Can you work these out from the model? Positions are in its coordinate system, mm. A direction names the side the tool comes from. Coordinates: 2 decimals unless noted, no trailing zeros. Loops run counter-clockwise (first coordinate to the right, second up) from the corner with the lowest first, then second, coordinate; pieces in that order, holes last.
```python
from build123d import *

# Parameters (mm, degrees)
SKETCH1_R           = 1.5
SKETCH1_R_2         = 18
BOSS_EXTRUDE1_DEPTH = 2
SKETCH1_3_R         = 31
SKETCH1_3_R_2       = 25
BOSS_EXTRUDE2_DEPTH = 1


with BuildPart() as part:
    # Sketch1 → Boss-Extrude1 (new body)
    with BuildSketch(Plane(origin=(0, 0, 0), x_dir=(1, 0, 0), z_dir=(0, 1, 0))):
        with BuildLine():
            ThreePointArc((33.442622951, 6.131147541), (24.04163056, 24.04163056), (6.131147541, 33.442622951))
            ThreePointArc((6.131147541, 33.442622951), (4.602624673, 34.335520561), (4, 36))
            ThreePointArc((4, 36), (0, 40), (-4, 36))
            ThreePointArc((-4, 36), (-4.602624673, 34.335520561), (-6.131147541, 33.442622951))
            ThreePointArc((-6.131147541, 33.442622951), (-24.04163056, 24.04163056), (-33.442622951, 6.131147541))
            ThreePointArc((-33.442622951, 6.131147541), (-34.335520561, 4.602624673), (-36, 4))
            ThreePointArc((-36, 4), (-40, 0), (-36, -4))
            ThreePointArc((-36, -4), (-34.335520561, -4.602624673), (-33.442622951, -6.131147541))
            ThreePointArc((-33.442622951, -6.131147541), (-24.04163056, -24.04163056), (-6.131147541, -33.442622951))
            ThreePointArc((-6.131147541, -33.442622951), (-4.602624673, -34.335520561), (-4, -36))
            ThreePointArc((-4, -36), (0, -40), (4, -36))
            ThreePointArc((4, -36), (4.602624673, -34.335520561), (6.131147541, -33.442622951))
            ThreePointArc((6.131147541, -33.442622951), (24.04163056, -24.04163056), (33.442622951, -6.131147541))
            ThreePointArc((33.442622951, -6.131147541), (34.335520561, -4.602624673), (36, -4))
            ThreePointArc((36, -4), (40, 0), (36, 4))
            ThreePointArc((36, 4), (34.335520561, 4.602624673), (33.442622951, 6.131147541))
        make_face()
        with Locations((36, 0)):
            Circle(SKETCH1_R, mode=Mode.SUBTRACT)
        with Locations((0, -36)):
            Circle(SKETCH1_R, mode=Mode.SUBTRACT)
        with Locations((0, 36)):
            Circle(SKETCH1_R, mode=Mode.SUBTRACT)
        with Locations((-36, 0)):
            Circle(SKETCH1_R, mode=Mode.SUBTRACT)
        Circle(SKETCH1_R_2, mode=Mode.SUBTRACT)
    extrude(amount=BOSS_EXTRUDE1_DEPTH)

    # Sketch1<3> → Boss-Extrude2 (add)
    with BuildSketch(Plane(origin=(0, 0, 0), x_dir=(1, 0, 0), z_dir=(0, 1, 0))):
        Circle(SKETCH1_3_R)
        Circle(SKETCH1_3_R_2, mode=Mode.SUBTRACT)
    extrude(amount=-BOSS_EXTRUDE2_DEPTH)


solid = part.part
```
(1) I want a section at D-D on z = -12. Write out the boundary of the cut face in (x, y).
Check values:
outline: (-31.81, 0) - (-28.58, 0) - (-28.58, -1) - (-21.93, -1) - (-21.93, 0) - (-13.42, 0) - (-13.42, 2) - (-31.81, 2) - close; (13.42, 0) - (21.93, 0) - (21.93, -1) - (28.58, -1) - (28.58, 0) - (31.81, 0) - (31.81, 2) - (13.42, 2) - close
(2) I'm going to push flat-ended pins straight in: pin 1 (1.5 mm diameter, centred on x = 17.5, y = 1.5, fed in from -Z); pin 2 (5 mm diameter, centred on x = 0, z = 36, fed in from -Y). Where does each tip first touch, or does it pass through?
Check values:
pin 1: stops at z = -29.59
pin 2: stops at y = 0
(3) I want a section at B-B on z = 0. Write out the boundary of the cut face in (x, y), then the cut area to 3 significant figures.
Check values:
outline: (-40, 0) - (-37.5, 0) - (-37.5, 2) - (-40, 2) - close; (-34.5, 0) - (-31, 0) - (-31, -1) - (-25, -1) - (-25, 0) - (-18, 0) - (-18, 2) - (-34.5, 2) - close; (18, 0) - (25, 0) - (25, -1) - (31, -1) - (31, 0) - (34.5, 0) - (34.5, 2) - (18, 2) - close; (37.5, 0) - (40, 0) - (40, 2) - (37.5, 2) - close
area: 88.0 mm2
(4) If I drill on probe 1 along Z at (x, y) = (0, 1.45); probe 2 along Z at (x, y) = (36, 0.65), over which ranges is the centre line in solid material (lowest first)?
Check values:
probe 1: z = -40 to -37.5, -34.5 to -18, 18 to 34.5, 37.5 to 40
probe 2: z = -4 to -1.5, 1.5 to 4
(5) I want a section at A-A on x = 0. Write out the boundary of the cut face in (y, z).
Check values:
outline: (-1, -31) - (0, -31) - (0, -34.5) - (2, -34.5) - (2, -18) - (0, -18) - (0, -25) - (-1, -25) - close; (-1, 25) - (0, 25) - (0, 18) - (2, 18) - (2, 34.5) - (0, 34.5) - (0, 31) - (-1, 31) - close; (0, -40) - (2, -40) - (2, -37.5) - (0, -37.5) - close; (0, 37.5) - (2, 37.5) - (2, 40) - (0, 40) - close
(6) I want a section at C-C on y = 1.1. Write out the boundary of the cut face in (x, z), then the cut area to 3 significant figures.
Check values:
outline: (-36, -4) arc R2.6 cw to (-33.44, -6.13) arc R34 ccw to (-6.13, -33.44) arc R2.6 cw to (-4, -36) arc R4 ccw to (4, -36) arc R2.6 cw to (6.13, -33.44) arc R34 ccw to (33.44, -6.13) arc R2.6 cw to (36, -4) arc R4 ccw to (36, 4) arc R2.6 cw to (33.44, 6.13) arc R34 ccw to (6.13, 33.44) arc R2.6 cw to (4, 36) arc R4 ccw to (-4, 36) arc R2.6 cw to (-6.13, 33.44) arc R34 ccw to (-33.44, 6.13) arc R2.6 cw to (-36, 4) arc R4 ccw to start; hole circle Ø3 at (-36, 0); hole circle Ø36 at (0, 0); hole circle Ø3 at (0, -36); hole circle Ø3 at (0, 36); hole circle Ø3 at (36, 0)
area: 2,760 mm2
(7) Which directions (+Z, -Z, +X, -X, +Y, -Y) give clear straight access to the entire face, cutting with the end or side of a thin tool? Please do faces 1 (the flat face through (11, 0, 16)), 2 (the flat face through (-0.6, 2, -18.3)).
Check values:
face 1: -Y
face 2: +Z, -Z, +X, -X, +Y
(8) If we mould it in two halves opening along X, with no side actions, what happens to faces 3 (the cylindrical face through (0, 1, -40)), 4 (the cylindrical face through (-0.325, 0.986, 37.464)), 5 (the cylindrical face through (34.316, 0.986, 4.619))? For each: released by +X, released by -X, zero draft, split by the parting line, or undercut.
Check values:
face 3: split by the parting line
face 4: undercut
face 5: released by +X
